Could you check a few things on this model? Use its own coordinates, in mm. A direction names the side the tool comes from. Round coordinates to 2 decimals unless told otherwise and drop trailing zeros. Loops run counter-clockwise (first coordinate to the right, second up) from the corner with the lowest first, then second, coordinate; pieces in that order, holes last. Notation, with made-up numbers: (27.5, 35) -> (75.5, 35) arc R23 cw to (75.5, 49) -> close; hole circle Ø6 at (23, 20). An arc over 180 degrees is marked (long way). Write each question's results on one line, items separated by ' | '. Start each with the question number.
1) Which directions (+Z, -Z, +X, -X, +Y, -Y) give clear straight access to the entire face, cutting with the end or side of a thin tool? Please do faces 4 (the flat face through (8, 44, -54)), 5 (the flat face through (40, 42, -85)).
2) We'd pull the mould along Z, two halves only. Please class faces 1 (the cylindrical face through (112.112, 35.896, -48.761)), 2 (the flat face through (20, 51, -39.409)), 3 (the flat face through (-32, 59, -32)): pulls with the +Z half, pulls with the -Z half, needs draft (parallel to the pull), parting line crosses it, or undercut.
3) For P1, Ø17.5, axis at y = 50, z = -28.5, coming from the +X side; P2, Ø14.5, axis at y = 42.5, z = 3.5, coming from the -X side; P3, Ø8, axis at x = -29.5, y = 89.5, coming from the +Z side; P4, Ø6, axis at x = -95.5, z = -24.5, coming from the -Y side, each with a flat end and sliding along its axis, tell me the tip position at first contact or that it passes through.
4) Imagine slicing it at D-D, the plane z = -93.5. List the corners of the cut face in (x, y) for me.
5) Imagine slicing it at B-B, the plane x = 0. List the corners of the cut face in (y, z) for me, plus the area to 3 significant figures.
6) Imagine slicing it at A-A, the plane z = 10. List the corners of the cut face in (x, y) for me, plus the area to 3 significant figures.
7) Imagine slicing it at C-C, the plane y = 96.5. List the corners of the cut face in (x, z) for me, plus the area to 3 significant figures.
8) If I drill on probe 1 along X at (y, z) = (30, -64); probe 2 along X at (y, z) = (17, 30); probe 3 along Y at (x, z) = (0, -33.5), over which ranges is the centre line in solid material (lowest first)?
from build123d import *

# Parameters (mm, degrees)
SKETCH_3_R               = 24
SKETCH_3_R_2             = 12
EXTRUDE_2_DEPTH          = 20
SKETCH_3_7_R             = 24
SKETCH_3_7_R_2           = 12
EXTRUDE_3_DEPTH          = 26
SKETCH_10_R              = 32
SKETCH_10_R_2            = 16
EXTRUDE_5_DEPTH          = 100
EXTRUDE_6_REACH          = 180.449
EXTRUDE_6_END_RADIUS     = 32
SKETCH_15_W              = 16
SKETCH_15_H              = 100
EXTRUDE_9_REACH          = 180.449
EXTRUDE_9_END_RADIUS     = 32
SKETCH_25_R              = 32
SKETCH_25_R_2            = 16
EXTRUDE_10_DEPTH         = 128
CUT_EXTRUDE_1_DEPTH      = 231.628319156
CUT_EXTRUDE_1_DEPTH_BACK = 231.628319156
SKETCH_28_R              = 10
EXTRUDE_11_DEPTH         = 16
EXTRUDE_12_DEPTH         = 16
EXTRUDE_13_REACH         = 228.769
EXTRUDE_13_END_RADIUS    = 32
EXTRUDE_14_REACH         = 228.769
EXTRUDE_14_END_RADIUS    = 32
SKETCH_38_W              = 16
SKETCH_38_H              = 22


with BuildPart() as part:
    # Sketch 3 → Extrude 2 (new body)
    # profile 1 of 4: a face of its own
    with BuildSketch(Plane(origin=(0, 0, 0), x_dir=(1, 0, 0), z_dir=(0, 1, 0))):
        with BuildLine():
            ThreePointArc((-120, 30), (-108.284271247, 58.284271247), (-80, 70))
            Line((-80, 70), (120, 70))
            Line((120, 70), (120, -30))
            ThreePointArc((120, -30), (108.284271247, -58.284271247), (80, -70))
            Line((80, -70), (-80, -70))
            ThreePointArc((-80, -70), (-108.284271247, -58.284271247), (-120, -30))
            Line((-120, -30), (-120, 30))
        make_face()
        with Locations((80, -10)):
            Circle(SKETCH_3_R, mode=Mode.SUBTRACT)
        with Locations((-80, -30)):
            Circle(SKETCH_3_R, mode=Mode.SUBTRACT)
        with Locations((-80, 30)):
            Circle(SKETCH_3_R, mode=Mode.SUBTRACT)
    # profile 2 of 4: a face of its own
    with BuildSketch(Plane(origin=(0, 0, 0), x_dir=(1, 0, 0), z_dir=(0, 1, 0))):
        with Locations((-80, -30)):
            Circle(SKETCH_3_R)
        with Locations(Location((-80, -30, 0), (0, 0, 270))):
            Circle(SKETCH_3_R_2, mode=Mode.SUBTRACT)
    # profile 3 of 4: a face of its own
    with BuildSketch(Plane(origin=(0, 0, 0), x_dir=(1, 0, 0), z_dir=(0, 1, 0))):
        with Locations((80, -10)):
            Circle(SKETCH_3_R)
        with Locations(Location((80, -10, 0), (0, 0, 270))):
            Circle(SKETCH_3_R_2, mode=Mode.SUBTRACT)
    # profile 4 of 4: a face of its own
    with BuildSketch(Plane(origin=(0, 0, 0), x_dir=(1, 0, 0), z_dir=(0, 1, 0))):
        with Locations((-80, 30)):
            Circle(SKETCH_3_R)
        with Locations(Location((-80, 30, 0), (0, 0, 270))):
            Circle(SKETCH_3_R_2, mode=Mode.SUBTRACT)
    extrude(amount=EXTRUDE_2_DEPTH)

    # Sketch 3_7 → Extrude 3 (add)
    # profile 1 of 3: a face of its own
    with BuildSketch(Plane(origin=(0, 0, 0), x_dir=(1, 0, 0), z_dir=(0, 1, 0))):
        with Locations(Location((-80, 30, 0), (0, 0, 90))):
            Circle(SKETCH_3_7_R)
        with Locations(Location((-80, 30, 0), (0, 0, 270))):
            Circle(SKETCH_3_7_R_2, mode=Mode.SUBTRACT)
    # profile 2 of 3: a face of its own
    with BuildSketch(Plane(origin=(0, 0, 0), x_dir=(1, 0, 0), z_dir=(0, 1, 0))):
        with Locations(Location((-80, -30, 0), (0, 0, 90))):
            Circle(SKETCH_3_7_R)
        with Locations(Location((-80, -30, 0), (0, 0, 270))):
            Circle(SKETCH_3_7_R_2, mode=Mode.SUBTRACT)
    # profile 3 of 3: a face of its own
    with BuildSketch(Plane(origin=(0, 0, 0), x_dir=(1, 0, 0), z_dir=(0, 1, 0))):
        with Locations(Location((80, -10, 0), (0, 0, 90))):
            Circle(SKETCH_3_7_R)
        with Locations(Location((80, -10, 0), (0, 0, 270))):
            Circle(SKETCH_3_7_R_2, mode=Mode.SUBTRACT)
    extrude(amount=EXTRUDE_3_DEPTH)



with BuildPart() as body_2:
    # Sketch 10 → Extrude 5 (new body)
    with BuildSketch(Plane(origin=(0, 0, -70), x_dir=(-1, 0, 0), z_dir=(0, 0, -1))):
        with Locations((0, 100)):
            Circle(SKETCH_10_R)
        with Locations((0, 100)):
            Circle(SKETCH_10_R_2, mode=Mode.SUBTRACT)
    extrude(amount=-EXTRUDE_5_DEPTH)


with BuildPart() as part_1:
    add(part.part)

    add(body_2.part)  # Extrude 6 merges body 2
    # Extrude 6: up to this cylinder (the profile starts outside it)
    extrude_6_end = Plane(origin=(0, 100, -20), z_dir=(0, 0, -1)) * Cylinder(EXTRUDE_6_END_RADIUS, 425.898, mode=Mode.PRIVATE)
    # Sketch 15 → Extrude 6 (add, up to the surface)
    with BuildSketch(Plane(origin=(0, 20, 0), x_dir=(1, 0, 0), z_dir=(0, 1, 0)), mode=Mode.PRIVATE) as extrude_6_sk1:
        with Locations((0, 20)):
            Rectangle(SKETCH_15_W, SKETCH_15_H)
    extrude_6_tool1 = extrude(extrude_6_sk1.sketch, amount=EXTRUDE_6_REACH, mode=Mode.PRIVATE) - extrude_6_end
    add(extrude_6_tool1.solids().sort_by_distance((0, 20, -20))[0])

    # Extrude 9: up to this cylinder (the profile starts outside it)
    extrude_9_end = Plane(origin=(0, 100, -31.409304), z_dir=(0, 0, -1)) * Cylinder(EXTRUDE_9_END_RADIUS, 425.898, mode=Mode.PRIVATE)
    # Sketch 16 → Extrude 9 (add, up to the surface)
    with BuildSketch(Plane(origin=(0, 20, 0), x_dir=(1, 0, 0), z_dir=(0, 1, 0)), mode=Mode.PRIVATE) as extrude_9_sk1:
        Polygon((32, 31.409304245), (32, 39.409304245), (8, 39.409304245), (8, 23.409304245), (32, 23.409304245), align=None)
    extrude_9_tool1 = extrude(extrude_9_sk1.sketch, amount=EXTRUDE_9_REACH, mode=Mode.PRIVATE) - extrude_9_end
    add(extrude_9_tool1.solids().sort_by_distance((20, 20, -31.409304))[0])
    # Sketch 16 → Extrude 9 (add, up to the surface)
    with BuildSketch(Plane(origin=(0, 20, 0), x_dir=(1, 0, 0), z_dir=(0, 1, 0)), mode=Mode.PRIVATE) as extrude_9_sk2:
        Polygon((-8, 23.409304245), (-8, 39.409304245), (-32, 39.409304245), (-32, 31.409304245), (-32, 23.409304245), align=None)
    extrude_9_tool2 = extrude(extrude_9_sk2.sketch, amount=EXTRUDE_9_REACH, mode=Mode.PRIVATE) - extrude_9_end
    add(extrude_9_tool2.solids().sort_by_distance((-20, 20, -31.409304))[0])

    # Sketch 30 → Extrude 11 (add)
    with BuildSketch(Plane(origin=(120, 0, 0), x_dir=(0, 0, -1), z_dir=(1, 0, 0))):
        with BuildLine():
            Line((70, 42), (70, 20))
            Line((70, 20), (34.278857801, 20))
            ThreePointArc((34.278857801, 20), (49.023823037, 36.058772732), (70, 42))
        make_face()
    extrude(amount=-EXTRUDE_11_DEPTH)

    # Sketch 34 → Extrude 12 (add)
    with BuildSketch(Plane(origin=(48, 0, 0), x_dir=(0, 0, -1), z_dir=(1, 0, 0))):
        with BuildLine():
            ThreePointArc((34.278857801, 20), (49.023823037, 36.058772732), (70, 42))
            Line((70, 42), (70, 20))
            Line((70, 20), (34.278857801, 20))
        make_face()
    extrude(amount=-EXTRUDE_12_DEPTH)



with BuildPart() as body_2_2:
    # Sketch 25 → Extrude 10 (new body)
    with BuildSketch(Plane(origin=(120, 0, 0), x_dir=(0, 0, -1), z_dir=(1, 0, 0))):
        with Locations(Location((130.004387585, 32, 0), (0, 0, 90))):
            Circle(SKETCH_25_R)
        with Locations(Location((130.004387585, 32, 0), (0, 0, 90))):
            Circle(SKETCH_25_R_2, mode=Mode.SUBTRACT)
    extrude(amount=-EXTRUDE_10_DEPTH)

    # Sketch 28 → Cut-Extrude 1 (cut, two sides: drawn at the far end of the back side and taken through both)
    with BuildSketch(Plane(origin=(0, 20, 0), x_dir=(1, 0, 0), z_dir=(0, 1, 0)).offset(-CUT_EXTRUDE_1_DEPTH_BACK)):
        with Locations(Location((56, 130.004387585, 0), (0, 0, 270))):
            Circle(SKETCH_28_R)
    extrude(amount=CUT_EXTRUDE_1_DEPTH + CUT_EXTRUDE_1_DEPTH_BACK, mode=Mode.SUBTRACT)


with BuildPart() as part_2:
    add(part_1.part)

    add(body_2_2.part)  # Extrude 13 merges body 2 2
    # Extrude 13: up to this cylinder (the profile starts outside it)
    extrude_13_end = Plane(origin=(111.937984, 32, -130.004387585), z_dir=(1, 0, 0)) * Cylinder(EXTRUDE_13_END_RADIUS, 522.538, mode=Mode.PRIVATE)
    # Sketch 37 → Extrude 13 (add, up to the surface)
    with BuildSketch(Plane(origin=(0, 0, -70), x_dir=(-1, 0, 0), z_dir=(0, 0, -1)), mode=Mode.PRIVATE) as extrude_13_sk1:
        Polygon((-104, 20), (-120, 21), (-120, 42), (-104, 42), align=None)
    extrude_13_tool1 = extrude(extrude_13_sk1.sketch, amount=EXTRUDE_13_REACH, mode=Mode.PRIVATE) - extrude_13_end
    add(extrude_13_tool1.solids().sort_by_distance((111.937984, 31.248062, -70))[0])

    # Extrude 14: up to this cylinder (the profile starts outside it)
    extrude_14_end = Plane(origin=(40, 32, -130.004387585), z_dir=(1, 0, 0)) * Cylinder(EXTRUDE_14_END_RADIUS, 522.538, mode=Mode.PRIVATE)
    # Sketch 38 → Extrude 14 (add, up to the surface)
    with BuildSketch(Plane(origin=(0, 0, -70), x_dir=(-1, 0, 0), z_dir=(0, 0, -1)), mode=Mode.PRIVATE) as extrude_14_sk1:
        with Locations((-40, 31)):
            Rectangle(SKETCH_38_W, SKETCH_38_H)
    extrude_14_tool1 = extrude(extrude_14_sk1.sketch, amount=EXTRUDE_14_REACH, mode=Mode.PRIVATE) - extrude_14_end
    add(extrude_14_tool1.solids().sort_by_distance((40, 31, -70))[0])


solid = part_2.part
Checked values:
1) face 4: none | face 5: +Z, +X, -X, +Y
2) face 1: pulls with the +Z half | face 2: undercut | face 3: needs draft
3) P1: x = 32 | P2: x = -8 | P3: z = 30 | P4: y = 0
4) outline: (32, 20) -> (48, 20) -> (48, 42) -> (32, 42) -> close; (104, 20) -> (120, 21) -> (120, 42) -> (104, 42) -> close
5) outline: circle Ø64 at (32, -130); (0, -70) -> (84, -70) -> (84, 30) -> (20, 30) -> (20, 70) -> (0, 70) -> close; (116, -70) -> (132, -70) -> (132, 30) -> (116, 30) -> close; hole circle Ø32 at (32, -130) | area: 13,200 mm^2
6) outline: (-120, 0) -> (68, 0) -> (68, 26) -> (56, 26) -> (56, 20) -> (8, 20) -> (8, 69.02) arc R32 ccw (long way) to (-8, 69.02) -> (-8, 20) -> (-66.73, 20) -> (-66.73, 26) -> (-93.27, 26) -> (-93.27, 20) -> (-120, 20) -> close; (92, 0) -> (120, 0) -> (120, 20) -> (104, 20) -> (104, 26) -> (92, 26) -> close; hole circle Ø32 at (0, 100) | area: 7,810 mm^2
7) outline: (-32, -39.41) -> (-31.81, -39.41) -> (-31.81, -70) -> (-15.61, -70) -> (-15.61, 30) -> (-31.81, 30) -> (-31.81, -23.41) -> (-32, -23.41) -> close; (15.61, -70) -> (31.81, -70) -> (31.81, -39.41) -> (32, -39.41) -> (32, -23.41) -> (31.81, -23.41) -> (31.81, 30) -> (15.61, 30) -> close | area: 3,250 mm^2
8) probe 1: -8 to 8, 32 to 48, 104 to 120 | probe 2: -120 to -92, -68 to 120 | probe 3: 0 to 84, 116 to 132
